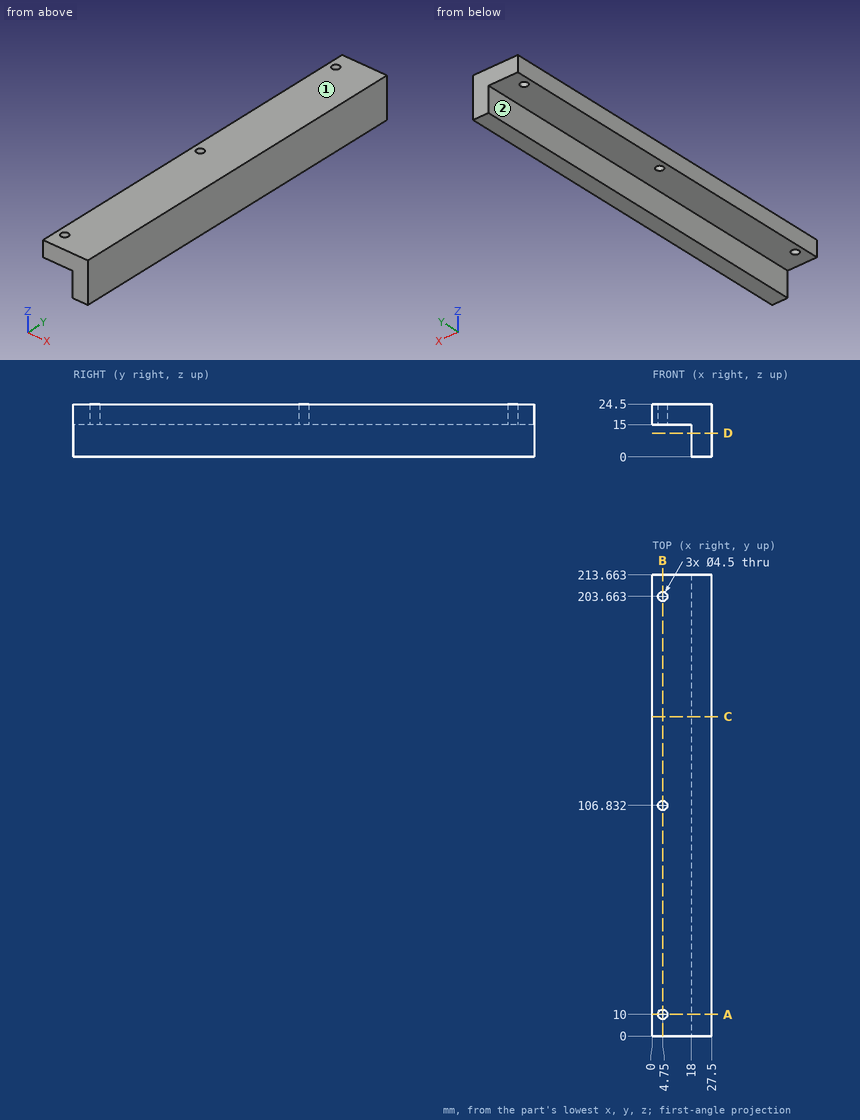
Drawing for the job (mm, zero at the part's lowest x, y, z). A direction names the side the tool comes from. Give positions to 0.01 mm unless a question says otherwise; leave off trailing zeros. Order: outer loops, then holes, each group sorted by start corner. A loop starts at its lowest first (then second) coordinate and runs counter-clockwise, first axis right, second up. Notation, with made-up numbers: M 68,46 L 98,46 A24 cw 98,69 Z; hole C 22.5,-28 d7. An arc over 180 degrees is marked long. Put each result on its own line as item: value.
Item 1: Slice it at B-B, the plane x = 4.75. Write the cut outline in (y, z).
From the geometry:
outline: M 0,15 L 7.75,15 L 7.75,24.5 L 0,24.5 Z; M 12.25,15 L 104.58,15 L 104.58,24.5 L 12.25,24.5 Z; M 109.08,15 L 201.41,15 L 201.41,24.5 L 109.08,24.5 Z; M 205.91,15 L 213.66,15 L 213.66,24.5 L 205.91,24.5 Z
Item 2: Slice it at A-A, the plane y = 10. Write the cut outline in (x, z), plus the area to 3 significant figures.
From the geometry:
outline: M 0,15 L 2.5,15 L 2.5,24.5 L 0,24.5 Z; M 7,15 L 18,15 L 18,0 L 27.5,0 L 27.5,24.5 L 7,24.5 Z
area: 361 mm2
Item 3: Flat gauge pins, fed straight in: pin 1 Ø2 at (y, z) = (135.5, 8.5) entering from -X; pin 2 Ø3.5 at (x, y) = (4.75, 10) entering from -Z; pin 3 Ø9 at (x, y) = (8.5, 116) entering from -Z. Where does each tip first touch, or does it go through?
From the geometry:
pin 1: stops at x = 18
pin 2: passes through
pin 3: stops at z = 15
Item 4: Slice it at D-D, the plane z = 11. Write the cut outline in (x, y).
From the geometry:
outline: M 18,0 L 27.5,0 L 27.5,213.66 L 18,213.66 Z
Item 5: Probe line 1 (Y direction, x = 4.75, z = 21.75); line 2 (X direction, y = 10, z = 20.5); line 3 (X direction, y = 184, z = 3). List the from-to ranges inside material, lowest first. Write a range as [from, to].
From the geometry:
line 1: y = [0, 7.75], [12.25, 104.58], [109.08, 201.41], [205.91, 213.66]
line 2: x = [0, 2.5], [7, 27.5]
line 3: x = [18, 27.5]
Item 6: Slice it at C-C, the plane y = 148. Write the cut outline in (x, z), plus the area to 3 significant figures.
From the geometry:
outline: M 0,15 L 18,15 L 18,0 L 27.5,0 L 27.5,24.5 L 0,24.5 Z
area: 404 mm2
Item 7: 3-axis set-ups, long thin cutter, end or side, ignore diameter. For the marked faces 1 and 2: which of +Z, -Z, +X, -X, +Y, -Y reach the whole face in a straight line?
From the geometry:
face 1: +Z, +X, -X, +Y, -Y
face 2: -Z, -X, +Y, -Y
